Work out the finished part from the listing and answer in its coordinate system (mm). A direction names the side the tool comes from. Coordinates: 2 decimals unless noted, no trailing zeros. Write each loop counter-clockwise with the first axis right and the second up, starting at its lowest first coordinate (ties: lowest second). Pieces come first, ordered by that corner, then holes. Notation, with made-up numbers: (41.5, 28.5) - (51.5, 28.5) arc R10 cw to (51.5, 43.5) - close; hole circle Ø9 at (25.25, 42). An arc over 180 degrees is marked (long way). Use a Markdown table: item, result. Add a question column.
(1) Given pin 1 Ø6 at (x, z) = (42, 18) entering from +Y; pin 2 Ø0.6 at (y, z) = (2, 18) entering from -X; pin 3 Ø2 at (x, y) = (98.5, 24) entering from +Z, each flat-ended and moving along its own axis, determine where each tip first touches the part or whether it passes through.
(2) The part is cut by section A-A, the plane x = 50.5. Give the vertices of the cut face in (y, z).
(3) The part is cut by section C-C, the plane z = 10. Give the vertices of the cut face in (x, y), then the cut area to 3 significant figures.
(4) Find the intervals of material crossed by line 1 (Z direction, x = 21.5, y = -2); line 2 (Y direction, x = 86, z = 19); line 3 (X direction, y = -4.5, z = 25.5), in increasing order. Write a range as from..to.
(5) The part is cut by section B-B, the plane y = 16.5. Give the vertices of the cut face in (x, z).
(6) The part is cut by section D-D, the plane x = 84.5. Give the vertices of the cut face in (y, z).
(7) For a pull along Y with two mould halves and no side action, classify faces 1 (the face through (5.45, 0.25, 0.99)), 2 (the face through (33.48, 16.89, 14.79)), 3 (the face through (21, 0.68, 13)), 4 (the face through (54.322, 34, 13)) as released by +Y, released by -Y, zero draft, split by the parting line, or undercut.
(8) A tool of negligible diameter and unlimited length cuts with its end or side. For faces 5 (the face through (86, 0.999, 13)), 6 (the face through (52.644, -31, 13)), 7 (the face through (86, 2.999, 13)), from which of +Z, -Z, +X, -X, +Y, -Y can it reach the whole face along a straight path? Write none if from no direction.
Autodesk Fusion 360 part; units mm, degrees
sketch "Boceto1" plane through (0, 0, 0) normal (0, 0, 1) x (1, 0, 0)
  circle A0 centre (53.322, 1.6797) radius 25
  circle A1 centre (53.322, 1.6797) radius 30
  line L0 (53.322, 36.6797) -> (113.322, 36.6797)
  line L1 (74.1438, -33.3203) -> (-6.3562, -33.3203)
  line L2 (-6.3562, -33.3203) -> (-6.678, 36.6797)
  line L3 (53.322, 36.6797) -> (-6.678, 36.6797)
  line L4 (53.322, 1.6797) -> (53.322, 36.6797)
  line L5 (113.322, 36.6797) -> (113.322, -33.3203)
  line L6 (113.322, -33.3203) -> (74.1438, -33.3203)
  line L7 (53.322, 31.6797) -> (54.322, 31.6797)
  line L8 (54.322, 31.6797) -> (54.322, 36.6797)
  line L9 (53.322, 31.6797) -> (52.322, 31.6797)
  line L10 (52.322, 31.6797) -> (52.322, 36.6797)
  line L11 (53.6438, -28.3186) -> (54.6438, -28.3186)
  line L12 (54.6438, -28.3186) -> (54.6438, -33.3203)
  line L13 (54.6438, -33.3203) -> (52.6438, -33.3203)
  line L14 (52.6438, -28.3127) -> (52.6438, -33.3203)
  line L15 (83.3203, 1.9993) -> (83.3203, 2.9993)
  line L16 (83.3203, 2.9993) -> (88.3203, 2.9993)
  line L17 (88.3203, 2.9993) -> (88.3203, 0.9993)
  line L18 (88.3203, 0.9993) -> (83.3143, 0.9993)
  line L19 (23.322, 1.6797) -> (18.322, 1.6797)
  line L20 (18.322, 1.6797) -> (18.322, 2.6797)
  line L21 (18.322, 2.6797) -> (23.3386, 2.6797)
  line L22 (18.322, 1.6797) -> (18.322, 0.6797)
  line L23 (18.322, 0.6797) -> (23.3386, 0.6797)
  dimension "d1" = 50
  dimension "d2" = 60
  dimension "d4" = 60
  dimension "d5" = 60
  dimension "d6" = 80.5
  dimension "d7" = 70
  dimension "d16" = 35
  dimension "d28" = 1
  dimension "d29" = 1
  dimension "d32" = 1
  dimension "d33" = 2
  dimension "d34" = 1
  dimension "d35" = 5
  dimension "d36" = 2
  dimension "d37" = 5
  dimension "d38" = 1
  dimension "d39" = 1
extrude "Extruir1" add sketch "Boceto1" along normal blind 30 contours A1 makes body 1
sketch "Boceto4" plane through (0, 0, 0) normal (0, 0, 1) x (1, 0, 0)
extrude "Extruir7" add sketch "Boceto1" along normal blind 25 separate body contours L3 L4 L9 L10 | L0 L4 L7 L8 makes body 2
extrude "Extruir8" add sketch "Boceto1" along normal blind 25 contours A1 L15 L16 L17 L18 | A1 L19 L20 L21 | A1 L19 L22 L23 | A1 L1 L11 L12 L13 L14 bodies 1
extrude "Extruir9" add sketch "Boceto1" along normal blind 2 contours A1 L1 L2 L3 L9 L10 L14 L20 L21 L22 L23 | A1 L0 L1 L5 L6 L7 L8 L11 L12 L15 L16 L17 L18 bodies 1 2
sketch "Boceto6" plane through (0, 0, 2) normal (0, 0, 1) x (-1, 0, 0)
  line L0 (-18.322, -0.6797) -> (-18.322, -2.6797)
  line L1 (-18.322, -2.6797) -> (-23.3386, -2.6797)
  arc A0 (-53.322, -31.6797) -> (-23.3386, -2.6797) centre (-53.322, -1.6797) ccw
  line L2 (-53.322, -31.6797) -> (-52.322, -31.6797)
  line L3 (-52.322, -31.6797) -> (-52.322, -36.6797)
  line L4 (-52.322, -36.6797) -> (6.678, -36.6797)
  line L5 (6.678, -36.6797) -> (6.3562, 33.3203)
  line L6 (6.3562, 33.3203) -> (-52.6438, 33.3203)
  line L7 (-52.6438, 33.3203) -> (-52.6438, 28.3127)
  arc A1 (-23.3386, -0.6797) -> (-52.6438, 28.3127) centre (-53.322, -1.6797) ccw
  line L8 (-23.3386, -0.6797) -> (-18.322, -0.6797)
  line L9 (-18.322, -1.6797) -> (6.5171, -1.6797)
  circle A2 centre (-5.9024, -1.6797) radius 2.5
  line L10 (-88.3203, -2.9993) -> (-88.3203, -0.9993)
  line L11 (-113.322, 33.3203) -> (-113.322, -36.6797)
  line L12 (-88.3203, -1.9993) -> (-113.322, -1.9993)
  circle A3 centre (-100.8211, -1.9993) radius 2.5
  point P0 (-18.322, -1.6797)
  dimension "d44" = 5
  dimension "d45" = 5
hole "Agujero2" at (100.8211, 1.9993, 2) direction (0, 0, -1) diameter 3 depth 10 tip angle 180 bodies 1
hole "Agujero3" at (5.9024, 1.6797, 2) direction (0, 0, -1) diameter 3 depth 10 tip angle 180 bodies 1
equation "d6 = 60 mm + 20.5 mm"
Model answer:
| question | item | result |
|---|---|---|
| 1 | pin 1 | y = 30.5 |
| 1 | pin 2 | x = 18.32 |
| 1 | pin 3 | z = 2 |
| 2 | outline | (-33.32, 0) - (-23.16, 0) - (-23.16, 30) - (-28.19, 30) - (-28.19, 2) - (-33.32, 2) - close; (26.52, 0) - (36.68, 0) - (36.68, 2) - (31.55, 2) - (31.55, 30) - (26.52, 30) - close |
| 3 | outline | (18.32, 0.68) - (23.34, 0.68) arc R30 ccw to (52.64, -28.31) - (52.64, -33.32) - (54.64, -33.32) - (54.64, -28.32) - (53.64, -28.32) arc R30 ccw to (83.31, 1) - (88.32, 1) - (88.32, 3) - (83.32, 3) - (83.32, 2) arc R30 ccw to (23.34, 2.68) - (18.32, 2.68) - close; (52.32, 31.68) - (54.32, 31.68) - (54.32, 36.68) - (52.32, 36.68) - close; hole circle Ø50 at (53.32, 1.68) |
| 3 | area | 904 mm^2 |
| 4 | line 1 | 0..2 |
| 4 | line 2 | 1..3 |
| 4 | line 3 | 23.97..29.1, 77.55..82.68 |
| 5 | outline | (-6.59, 0) - (33.19, 0) - (33.19, 30) - (27.24, 30) - (27.24, 2) - (-6.59, 2) - close; (73.46, 0) - (113.32, 0) - (113.32, 2) - (79.41, 2) - (79.41, 30) - (73.46, 30) - close |
| 6 | outline | (-33.32, 0) - (36.68, 0) - (36.68, 2) - (3, 2) - (3, 25) - (1, 25) - (1, 2) - (-33.32, 2) - close |
| 7 | face 1 | undercut |
| 7 | face 2 | undercut |
| 7 | face 3 | released by -Y |
| 7 | face 4 | zero draft |
| 8 | face 5 | +Z, +X, -Y |
| 8 | face 6 | +Z, -X, -Y |
| 8 | face 7 | +Z, +X, +Y |
